Part model, mm, in its own coordinate system. Give positions to 0.01 mm unless a question says otherwise; leave off trailing zeros. Write each loop counter-clockwise with the first axis right and the second up, starting at its lowest first coordinate (ties: lowest second). Pieces come first, ordered by that corner, then holes. Notation, with made-up numbers: M -7,54.5 L 44,54.5 A28 ccw 44,82.5 Z; hole C 70,44 d5. An arc over 180 degrees is marked long. Write item = value, one per line. Start each with the question number.
from build123d import *

# Parameters (mm, degrees)
SKETCH1_W           = 154
SKETCH1_H           = 60
BOSS_EXTRUDE1_DEPTH = 0.1
CUT_EXTRUDE1_DEPTH  = 83.63782427
SKETCH3_R           = 8
SKETCH3_W           = 154
SKETCH3_H           = 2
CUT_EXTRUDE2_DEPTH  = 0.05


with BuildPart() as part:
    # Sketch1 → Boss-Extrude1 (new body)
    with BuildSketch(Plane(origin=(0, 0, 0), x_dir=(1, 0, 0), z_dir=(0, 1, 0))):
        Rectangle(SKETCH1_W, SKETCH1_H)
    extrude(amount=BOSS_EXTRUDE1_DEPTH)

    # Sketch2 → Cut-Extrude1 (cut, through all)
    with BuildSketch(Plane(origin=(0, 0.1, 0), x_dir=(1, 0, 0), z_dir=(0, 1, 0))):
        with BuildLine():
            Line((51.2, 19.417618892), (51.2, 13.582381108))
            ThreePointArc((51.2, 13.582381108), (56.5, 10.45), (61.8, 13.582381108))
            Line((61.8, 13.582381108), (61.8, 19.417618892))
            ThreePointArc((61.8, 19.417618892), (56.5, 22.55), (51.2, 19.417618892))
        make_face()
        with BuildLine():
            Line((37.8, 19.417618892), (37.8, 13.582381108))
            ThreePointArc((37.8, 13.582381108), (32.5, 10.45), (27.2, 13.582381108))
            Line((27.2, 13.582381108), (27.2, 19.417618892))
            ThreePointArc((27.2, 19.417618892), (32.5, 22.55), (37.8, 19.417618892))
        make_face()
        with BuildLine():
            Line((13.8, 19.417618892), (13.8, 13.582381108))
            ThreePointArc((13.8, 13.582381108), (8.5, 10.45), (3.2, 13.582381108))
            Line((3.2, 13.582381108), (3.2, 19.417618892))
            ThreePointArc((3.2, 19.417618892), (8.5, 22.55), (13.8, 19.417618892))
        make_face()
        with BuildLine():
            Line((-10.2, 19.417618892), (-10.2, 13.582381108))
            ThreePointArc((-10.2, 13.582381108), (-15.5, 10.45), (-20.8, 13.582381108))
            Line((-20.8, 13.582381108), (-20.8, 19.417618892))
            ThreePointArc((-20.8, 19.417618892), (-15.5, 22.55), (-10.2, 19.417618892))
        make_face()
        with BuildLine():
            Line((-34.2, 19.417618892), (-34.2, 13.582381108))
            ThreePointArc((-34.2, 13.582381108), (-39.5, 10.45), (-44.8, 13.582381108))
            Line((-44.8, 13.582381108), (-44.8, 19.417618892))
            ThreePointArc((-44.8, 19.417618892), (-39.5, 22.55), (-34.2, 19.417618892))
        make_face()
        with BuildLine():
            Line((37.8, -5.582381108), (37.8, -11.417618892))
            ThreePointArc((37.8, -11.417618892), (32.5, -14.55), (27.2, -11.417618892))
            Line((27.2, -11.417618892), (27.2, -5.582381108))
            ThreePointArc((27.2, -5.582381108), (32.5, -2.45), (37.8, -5.582381108))
        make_face()
        with BuildLine():
            Line((13.8, -5.582381108), (13.8, -11.417618892))
            ThreePointArc((13.8, -11.417618892), (8.5, -14.55), (3.2, -11.417618892))
            Line((3.2, -11.417618892), (3.2, -5.582381108))
            ThreePointArc((3.2, -5.582381108), (8.5, -2.45), (13.8, -5.582381108))
        make_face()
        with BuildLine():
            Line((-10.2, -5.582381108), (-10.2, -11.417618892))
            ThreePointArc((-10.2, -11.417618892), (-15.5, -14.55), (-20.8, -11.417618892))
            Line((-20.8, -11.417618892), (-20.8, -5.582381108))
            ThreePointArc((-20.8, -5.582381108), (-15.5, -2.45), (-10.2, -5.582381108))
        make_face()
        with BuildLine():
            Line((-34.2, -5.582381108), (-34.2, -11.417618892))
            ThreePointArc((-34.2, -11.417618892), (-39.5, -14.55), (-44.8, -11.417618892))
            Line((-44.8, -11.417618892), (-44.8, -5.582381108))
            ThreePointArc((-44.8, -5.582381108), (-39.5, -2.45), (-34.2, -5.582381108))
        make_face()
        with BuildLine():
            Line((61.8, -5.582381108), (61.8, -11.417618892))
            ThreePointArc((61.8, -11.417618892), (56.5, -14.55), (51.2, -11.417618892))
            Line((51.2, -11.417618892), (51.2, -5.582381108))
            ThreePointArc((51.2, -5.582381108), (56.5, -2.45), (61.8, -5.582381108))
        make_face()
        with BuildLine():
            Line((-51.2, 6.917618892), (-51.2, 1.082381108))
            ThreePointArc((-51.2, 1.082381108), (-56.5, -2.05), (-61.8, 1.082381108))
            Line((-61.8, 1.082381108), (-61.8, 6.917618892))
            ThreePointArc((-61.8, 6.917618892), (-56.5, 10.05), (-51.2, 6.917618892))
        make_face()
    extrude(amount=-CUT_EXTRUDE1_DEPTH, mode=Mode.SUBTRACT)

    # Sketch3 → Cut-Extrude2 (cut)
    with BuildSketch(Plane(origin=(0, 0.1, 0), x_dir=(1, 0, 0), z_dir=(0, 1, 0))):
        with Locations(Location((-56.5, 4, 0), (0, 0, 270))):
            Circle(SKETCH3_R)
        with Locations(Location((56.5, 16.5, 0), (0, 0, 270))):
            Circle(SKETCH3_R)
        with Locations(Location((32.5, 16.5, 0), (0, 0, 270))):
            Circle(SKETCH3_R)
        with Locations(Location((8.5, 16.5, 0), (0, 0, 270))):
            Circle(SKETCH3_R)
        with Locations(Location((-15.5, 16.5, 0), (0, 0, 270))):
            Circle(SKETCH3_R)
        with Locations(Location((-39.5, 16.5, 0), (0, 0, 270))):
            Circle(SKETCH3_R)
        with Locations(Location((32.5, -8.5, 0), (0, 0, 270))):
            Circle(SKETCH3_R)
        with Locations(Location((8.5, -8.5, 0), (0, 0, 270))):
            Circle(SKETCH3_R)
        with Locations(Location((-15.5, -8.5, 0), (0, 0, 270))):
            Circle(SKETCH3_R)
        with Locations(Location((-39.5, -8.5, 0), (0, 0, 270))):
            Circle(SKETCH3_R)
        with Locations(Location((56.5, -8.5, 0), (0, 0, 270))):
            Circle(SKETCH3_R)
        with Locations((0, 29)):
            Rectangle(SKETCH3_W, SKETCH3_H)
    extrude(amount=-CUT_EXTRUDE2_DEPTH, mode=Mode.SUBTRACT)


solid = part.part
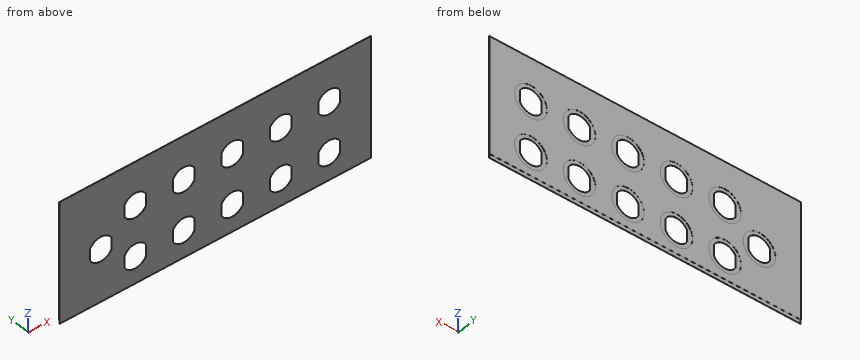
Q1. Drop a flat-ended pin along its axis: P1, Ø0.6, axis at x = 17.5, z = -29.5, coming from the +Y side. Give the stop position or say it passes through.
Q2. Slice it at C-C (z = -16.5). Give the number of separate pieces and of enclosed holes in the cut face, and give its area (3 significant figures).
Q3. Slice it at A-A (z = -4). Give the cut face in (x, y).
Q4. Slice it at B-B (x = -39.5). Give the cut face in (y, z).
Working result:
q1.P1 = 0.05
q2.separate_pieces = 6
q2.enclosed_holes = 0
q2.area = 8.75 mm2
q3.outline = M -77,0 L -61.8,0 L -61.8,0.05 L -64.5,0.05 L -64.5,0.1 L -77,0.1 Z; M -51.2,0 L 77,0 L 77,0.1 L -48.5,0.1 L -48.5,0.05 L -51.2,0.05 Z
q4.outline = M 0,-30 L 0.05,-30 L 0.05,-28 L 0.1,-28 L 0.1,-24.5 L 0.05,-24.5 L 0.05,-22.55 L 0,-22.55 Z; M 0,-10.45 L 0.05,-10.45 L 0.05,-8.5 L 0.1,-8.5 L 0.1,0.5 L 0.05,0.5 L 0.05,2.45 L 0,2.45 Z; M 0,14.55 L 0.05,14.55 L 0.05,16.5 L 0.1,16.5 L 0.1,30 L 0,30 Z
